```python
from build123d import *

# Parameters (mm, degrees)
SKETCH1_W           = 42.5
SKETCH1_H           = 42.5
BOSS_EXTRUDE1_DEPTH = 47
CHAMFER1_SIZE       = 5
SKETCH2_R           = 2.5
BOSS_EXTRUDE2_DEPTH = 24.5


with BuildPart() as part:
    # Sketch1 → Boss-Extrude1 (new body)
    with BuildSketch(Plane.XY):
        with Locations((-20.394847779, 6.347974521)):
            Rectangle(SKETCH1_W, SKETCH1_H)
    extrude(amount=BOSS_EXTRUDE1_DEPTH)

    # Chamfer1
    chamfer1_edges = [part.edges().sort_by_distance(p)[0] for p in [
        (-41.644847779, 27.597974521, 23.5),
        (0.855152221, 27.597974521, 23.5),
        (0.855152221, -14.902025479, 23.5),
        (-41.644847779, -14.902025479, 23.5),
    ]]
    chamfer(chamfer1_edges, length=CHAMFER1_SIZE)

    # Sketch2 → Boss-Extrude2 (add)
    with BuildSketch(Plane.XY.offset(47)):
        with Locations((-20.394847779, 6.347974521)):
            Circle(SKETCH2_R)
    extrude(amount=BOSS_EXTRUDE2_DEPTH)


solid = part.part
```
CAD build for the part. Positions are in the model's coordinates, mm. A direction names the side the tool comes from. Round coordinates to 2 decimals unless told otherwise and drop trailing zeros. Loops run counter-clockwise (first coordinate to the right, second up) from the corner with the lowest first, then second, coordinate; pieces in that order, holes last. Notation, with made-up numbers: M 43.25,22 L 48.25,22 A17 cw 48.25,29 Z; hole C -12,54.5 d1. An arc over 180 degrees is marked long. Use a Markdown table: item, result. Add a question column.
(1) Cut at B-B (x = -20). Give the cut face in (y, z), and give its area (3 significant figures).
(2) Cut at D-D (x = -15.5). Give the cut face in (y, z), and give its area (3 significant figures).
(3) Cut at A-A (z = 29.5). Give the cut face in (x, y).
(4) Cut at C-C (y = -6.5). Give the cut face in (x, z), and give its area (3 significant figures).
(5) Flat gauge pin, fed straight in: pin 1 (6 mm diameter, centred on x = -36, y = 11.5, fed in from +Z). Where does the tip first touch, or does it go through?
(6) Pull direction Y, two halves, no side cores. Call faces 3 (the face through (-20, 6, 71.5)), 4 (the face through (-39.11, -12.437, 23.171)), 5 (the face through (-21, 27.598, 23)): +Y half, -Y half, draft (parallel to the pull), parting line (faces both ways), or undercut.
(7) Which spindle directions (+Z, -Z, +X, -X, +Y, -Y) get a long thin tool onto all of the face, cutting with end or side? Do faces 1 (the face through (-22.892, 6.458, 59.078)), 2 (the face through (-41.645, 6, 23)). Say none if no direction does.
(8) Drill centre lines: line 1 (Z direction, x = -6, y = 9); line 2 (Y direction, x = -37, z = 5); line 3 (X direction, y = -12, z = 24). Where is each one in solid material? Low to high.
Geometry says:
| question | item | result |
|---|---|---|
| 1 | outline | M -14.9,0 L 27.6,0 L 27.6,47 L 8.82,47 L 8.82,71.5 L 3.88,71.5 L 3.88,47 L -14.9,47 Z |
| 1 | area | 2,120 mm² |
| 2 | outline | M -14.9,0 L 27.6,0 L 27.6,47 L -14.9,47 Z |
| 2 | area | 2,000 mm² |
| 3 | outline | M -41.64,-9.9 L -36.64,-14.9 L -4.14,-14.9 L 0.86,-9.9 L 0.86,22.6 L -4.14,27.6 L -36.64,27.6 L -41.64,22.6 Z |
| 4 | outline | M -41.64,0 L 0.86,0 L 0.86,47 L -41.64,47 Z |
| 4 | area | 2,000 mm² |
| 5 | pin 1 | stops at z = 47 |
| 6 | face 3 | draft |
| 6 | face 4 | -Y half |
| 6 | face 5 | +Y half |
| 7 | face 1 | +Z |
| 7 | face 2 | +Z, -Z, -X, +Y, -Y |
| 8 | line 1 | z = 0 to 47 |
| 8 | line 2 | y = -14.55 to 27.24 |
| 8 | line 3 | x = -39.55 to -1.24 |
